Build history of the part. All positions in model axes, mm. Give positions to 0.01 mm unless a question says otherwise; leave off trailing zeros. Write each loop counter-clockwise with the first axis right and the second up, starting at its lowest first coordinate (ties: lowest second). Pieces come first, ordered by that corner, then holes. Notation, with made-up numbers: (86, 28.25) -> (106, 28.25) arc R37 ccw to (106, 67.25) -> close; hole circle Ø5 at (-24, -16.75). An arc over 180 degrees is marked (long way). Put each result on its own line as item: value.
from build123d import *

# Parameters (mm, degrees)
ESQUISSE1_R             = 18.5
BOSS_EXTRU_1_DEPTH      = 5
ESQUISSE2_R             = 2
ENL_V_MAT_EXTRU_1_DEPTH = 6
ESQUISSE3_R             = 6.25
ENL_V_MAT_EXTRU_2_DEPTH = 6


with BuildPart() as part:
    # Esquisse1 → Boss.-Extru.1 (new body)
    with BuildSketch(Plane.XY):
        Circle(ESQUISSE1_R)
    extrude(amount=BOSS_EXTRU_1_DEPTH)

    # Esquisse2 → Enlèv. mat.-Extru.1 (cut, through all)
    with BuildSketch(Plane.XY.offset(5)):
        with Locations((-15.5, 0)):
            Circle(ESQUISSE2_R)
        with Locations((15.5, 0)):
            Circle(ESQUISSE2_R)
        with Locations((7.75, -13.423393759)):
            Circle(ESQUISSE2_R)
        with Locations((-7.75, -13.423393759)):
            Circle(ESQUISSE2_R)
        with Locations((-7.75, 13.423393759)):
            Circle(ESQUISSE2_R)
        with Locations((7.75, 13.423393759)):
            Circle(ESQUISSE2_R)
    extrude(amount=-ENL_V_MAT_EXTRU_1_DEPTH, mode=Mode.SUBTRACT)

    # Esquisse3 → Enlèv. mat.-Extru.2 (cut, through all)
    with BuildSketch(Plane.XY.offset(5)):
        with Locations((0, -7)):
            Circle(ESQUISSE3_R)
    extrude(amount=-ENL_V_MAT_EXTRU_2_DEPTH, mode=Mode.SUBTRACT)


solid = part.part
1) Slice it at C-C (x = -7.75). Write the cut outline in (y, z).
Filled sheet:
outline: (-16.8, 0) -> (-15.42, 0) -> (-15.42, 5) -> (-16.8, 5) -> close; (-11.42, 0) -> (11.42, 0) -> (11.42, 5) -> (-11.42, 5) -> close; (15.42, 0) -> (16.8, 0) -> (16.8, 5) -> (15.42, 5) -> close
2) Wall check: L1, parallel to X at y = 14, z = 1.2; L2, parallel to Y at x = 0, z = 1.1; L3, parallel to Y at x = 7.75, z = 2.8. Give the ranges that are in metal, low to high.
Filled sheet:
L1: -12.09 to -9.67, -5.83 to 5.83, 9.67 to 12.09
L2: -18.5 to -13.25, -0.75 to 18.5
L3: -16.8 to -15.42, -11.42 to 11.42, 15.42 to 16.8
3) Pin check, flat tips, straight feed: pin 1 (1 mm diameter, centred on x = -4, z = 1, fed in from -Y); pin 2 (2 mm diameter, centred on y = -8, z = 2, fed in from -X); pin 3 (3 mm diameter, centred on x = -7.75, y = -13.42, fed in from -Z). Stop position of each tip, or through.
Filled sheet:
pin 1: y = -18.17
pin 2: x = -17.12
pin 3: through
4) Slice it at A-A (y = 0). Write the cut outline in (x, z).
Filled sheet:
outline: (-18.5, 0) -> (-17.5, 0) -> (-17.5, 5) -> (-18.5, 5) -> close; (-13.5, 0) -> (13.5, 0) -> (13.5, 5) -> (-13.5, 5) -> close; (17.5, 0) -> (18.5, 0) -> (18.5, 5) -> (17.5, 5) -> close
5) Pull direction X, two halves, no side cores. Call faces 1 (the cylindrical face through (-4.01, -18.06, 2.46)), 2 (the flat face through (0, 0, 0)), 3 (the cylindrical face through (-9.75, -13.34, 2.54)): released by +X, released by -X, zero draft, split by the parting line, or undercut.
Filled sheet:
face 1: split by the parting line
face 2: zero draft
face 3: undercut
6) Slice it at B-B (x = 0). Write the cut outline in (y, z), plus the area to 4 significant figures.
Filled sheet:
outline: (-18.5, 0) -> (-13.25, 0) -> (-13.25, 5) -> (-18.5, 5) -> close; (-0.75, 0) -> (18.5, 0) -> (18.5, 5) -> (-0.75, 5) -> close
area: 122.5 mm2
7) Slice it at D-D (z = 3.8). Write the cut outline in (x, y), plus the area to 3 significant figures.
Filled sheet:
outline: circle Ø37 at (0, 0); hole circle Ø4 at (-15.5, 0); hole circle Ø4 at (-7.75, -13.42); hole circle Ø4 at (-7.75, 13.42); hole circle Ø12.5 at (0, -7); hole circle Ø4 at (7.75, -13.42); hole circle Ø4 at (7.75, 13.42); hole circle Ø4 at (15.5, 0)
area: 877 mm2
